Input: dimensioned drawing with shaded views. Units: mm. Origin: part minimum x, y, z. A direction names the side the tool comes from. Round coordinates to 2 decimals unless told otherwise and drop trailing zeros. Loops run counter-clockwise (first coordinate to the right, second up) from the corner with the lowest first, then second, coordinate; pieces in that order, holes last.
1) First-contact query: pin 1 (3 mm diameter, centred on x = 3, z = 10, fed in from +Y); pin 2 (1 mm diameter, centred on y = 0.5, z = 8.5, fed in from -X). Flat tips, straight axial feed; report the tip coordinate or a pass-through.
2) Access query for the marked faces 5 and 6. Directions: +Z, -Z, +X, -X, +Y, -Y. A direction counts if a zero-diameter tool reaches every point of the face in a straight line with its end or side. Return the directions, or none.
3) Ray query, line 1 along X through (y, z) = (0.6, 10); line 2 along X through (y, z) = (3.5, 10) (3 decimals). Return the intervals inside material, ascending.
4) Section A-A, the plane x = 10. Return loops of the section in (y, z) (3 decimals), and give its area (3 significant figures).
5) Section B-B, the plane z = 10. Return loops of the section in (x, y) (3 decimals), and give its area (3 significant figures).
6) Section D-D, the plane z = 17. Return loops of the section in (x, y).
7) Section C-C, the plane y = 2.9. Return loops of the section in (x, z) (3 decimals).
8) Draft query along X for the marked faces 1, 2, 3 and 4. Return one class per face: pulls with the +X half, pulls with the -X half, needs draft (parallel to the pull), parting line crosses it, or undercut.
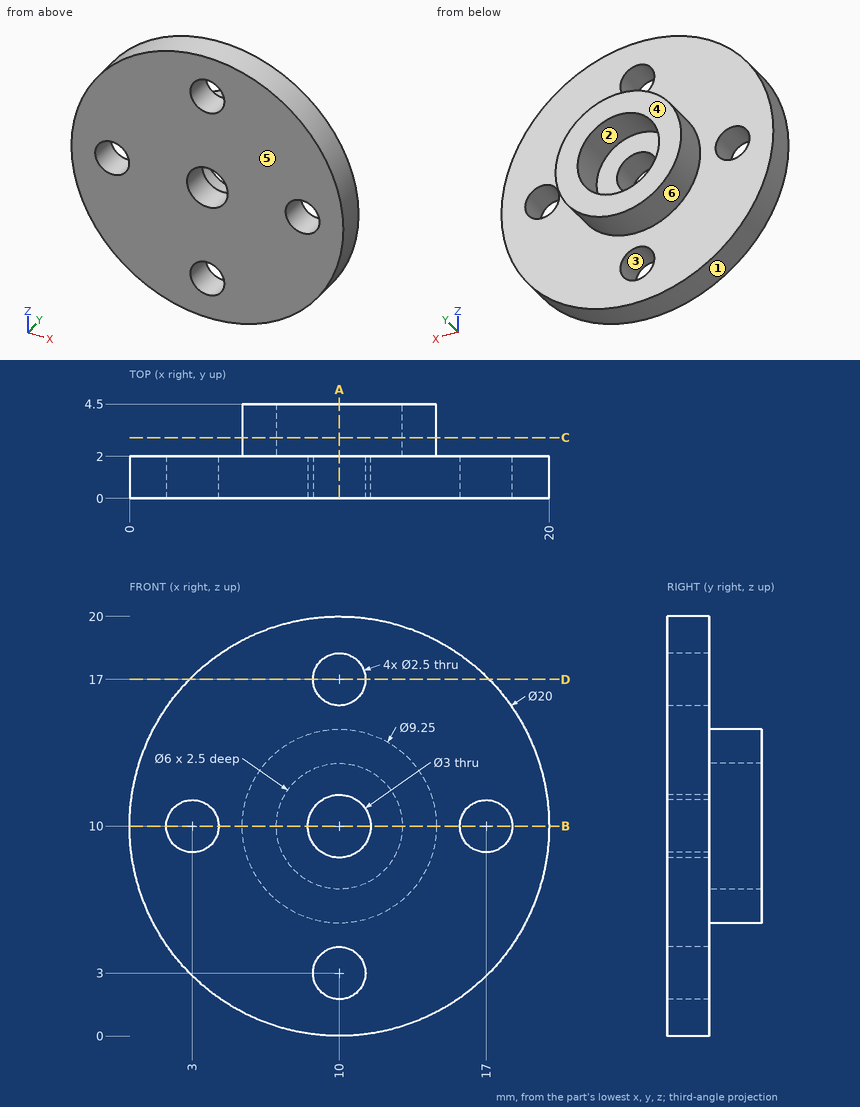
Final values:
1. pin 1: stops at y = 2
1. pin 2: stops at x = 0.05
2. face 5: +Z, -Z, +X, -X, -Y
2. face 6: +Y
3. line 1: x = 0 to 1.75, 4.25 to 8.5, 11.5 to 15.75, 18.25 to 20
3. line 2: x = 5.375 to 7, 13 to 14.625
4. outline: (0, 0) - (2, 0) - (2, 1.75) - (0, 1.75) - close; (0, 4.25) - (2, 4.25) - (2, 5.375) - (4.5, 5.375) - (4.5, 7) - (2, 7) - (2, 8.5) - (0, 8.5) - close; (0, 11.5) - (2, 11.5) - (2, 13) - (4.5, 13) - (4.5, 14.625) - (2, 14.625) - (2, 15.75) - (0, 15.75) - close; (0, 18.25) - (2, 18.25) - (2, 20) - (0, 20) - close
4. area: 32.1 mm2
5. outline: (0, 0) - (1.75, 0) - (1.75, 2) - (0, 2) - close; (4.25, 0) - (8.5, 0) - (8.5, 2) - (7, 2) - (7, 4.5) - (5.375, 4.5) - (5.375, 2) - (4.25, 2) - close; (11.5, 0) - (15.75, 0) - (15.75, 2) - (14.625, 2) - (14.625, 4.5) - (13, 4.5) - (13, 2) - (11.5, 2) - close; (18.25, 0) - (20, 0) - (20, 2) - (18.25, 2) - close
5. area: 32.1 mm2
6. outline: (2.86, 0) - (8.75, 0) - (8.75, 2) - (2.86, 2) - close; (11.25, 0) - (17.14, 0) - (17.14, 2) - (11.25, 2) - close
7. outline: circle Ø9.25 at (10, 10); hole circle Ø6 at (10, 10)
8. face 1: parting line crosses it
8. face 2: undercut
8. face 3: undercut
8. face 4: needs draft
